Design review of the part built by this model. Coordinates are the model's own, in mm. Coordinates: 2 decimals unless noted, no trailing zeros. Loops run counter-clockwise (first coordinate to the right, second up) from the corner with the lowest first, then second, coordinate; pieces in that order, holes last. Notation, with made-up numbers: M 10,-9.5 L 61,-9.5 A17 cw 61,19.5 Z; hole C 73.25,-29.5 d1. An arc over 180 degrees is marked long. One line per item, written item: value.
```python
from build123d import *

# Parameters (mm, degrees)
CYLINDER071_R     = 21
CYLINDER071_DEPTH = 2
CYLINDER070_R     = 24
CYLINDER070_DEPTH = 1.8


with BuildPart() as cylinder071:
    # Cylinder071 → Cylinder071 (new body)
    with BuildSketch(Plane.XY.offset(20)):
        Circle(CYLINDER071_R)
    extrude(amount=CYLINDER071_DEPTH)


with BuildPart() as rim_support:
    # Cylinder070 → Cylinder070 (new body)
    with BuildSketch(Plane.XY.offset(20)):
        Circle(CYLINDER070_R)
    extrude(amount=CYLINDER070_DEPTH)

    # Cut020: cut Cylinder071
    add(cylinder071.part, mode=Mode.SUBTRACT)


with BuildPart() as rim_support_1:
    # Cut020 placement: moved
    add(rim_support.part.moved(Location((0, 0, 0.2))))


solid = rim_support_1.part
```
(1) We need section C-C on z = 21.05. State the section outline as (x, y) points.
Reply:
outline: C 0,0 d48; hole C 0,0 d42
(2) We need section B-B on x = -15. State the section outline as (y, z) points (3 decimals).
Reply:
outline: M -18.735,20.2 L -14.697,20.2 L -14.697,22 L -18.735,22 Z; M 14.697,20.2 L 18.735,20.2 L 18.735,22 L 14.697,22 Z
(3) To check wall thickness, follow line 1 along Y through (x, z) = (0, 21.6); line 2 along Y through (x, z) = (2.5, 21.8); line 3 along X through (y, z) = (-5, 20.8). State the ranges of each line that lie inside material, in increasing order. Write a range as [from, to].
Reply:
line 1: y = [-24, -21], [21, 24]
line 2: y = [-23.87, -20.85], [20.85, 23.87]
line 3: x = [-23.47, -20.4], [20.4, 23.47]
(4) Mouldability with a two-part tool opening along X and no side actions: class faces 1 (the flat face through (-0.1, -21.2, 20.2)), 2 (the cylindrical face through (20.03, 6.31, 21.09)), 3 (the cylindrical face through (-23.977, 1.055, 21.087)) as released by +X, released by -X, zero draft, split by the parting line, or undercut.
Reply:
face 1: zero draft
face 2: undercut
face 3: split by the parting line
(5) We need section A-A on y = 0. State the section outline as (x, z) points.
Reply:
outline: M -24,20.2 L -21,20.2 L -21,22 L -24,22 Z; M 21,20.2 L 24,20.2 L 24,22 L 21,22 Z
(6) Insertion check: pin 1 (1 mm diameter, centred on y = 16, z = 21, fed in from +X). The pin has a flat end and moves straight along its axis. Give the tip position at first contact, or say it passes through.
Reply:
pin 1: stops at x = 18.32
